Geometry: final body of the model. Coordinates: model frame, mm. Coordinates: 2 decimals unless noted, no trailing zeros. Write each loop counter-clockwise with the first axis right and the second up, starting at its lowest first coordinate (ties: lowest second). Pieces come first, ordered by that corner, then holes.
from build123d import *

# Parameters (mm, degrees)
SKETCH1_W              = 263.525
SKETCH1_H              = 50.8
BOSS_EXTRUDE1_DEPTH    = 1.143
F_10_CLEARANCE_HOLE1_D = 5.1054


with BuildPart() as part:
    # Sketch1 → Boss-Extrude1 (new, symmetric)
    with BuildSketch(Plane.XY):
        Rectangle(SKETCH1_W, SKETCH1_H)
    extrude(amount=BOSS_EXTRUDE1_DEPTH, both=True)

    # #10 Clearance Hole1 (through all)
    with Locations(Plane.XY.offset(1.143)):
        with Locations((-119.0625, 12.7), (-119.0625, -12.7), (-12.7, 12.7), (-12.7, -12.7), (12.7, -12.7), (12.7, 12.7), (119.0625, 12.7), (119.0625, -12.7)):
            Hole(F_10_CLEARANCE_HOLE1_D / 2)


solid = part.part
Item 1: Section A-A, the plane y = -12.7. Output: boundary loops of the cut face in (x, z).
Derived:
outline: (-131.76, -1.14) - (-121.62, -1.14) - (-121.62, 1.14) - (-131.76, 1.14) - close; (-116.51, -1.14) - (-15.25, -1.14) - (-15.25, 1.14) - (-116.51, 1.14) - close; (-10.15, -1.14) - (10.15, -1.14) - (10.15, 1.14) - (-10.15, 1.14) - close; (15.25, -1.14) - (116.51, -1.14) - (116.51, 1.14) - (15.25, 1.14) - close; (121.62, -1.14) - (131.76, -1.14) - (131.76, 1.14) - (121.62, 1.14) - close
Item 2: Material intervals for probe 1 along Y at (x, z) = (12.7, -0.3); probe 2 along X at (y, z) = (-12, 0.55), sorted ascending.
Derived:
probe 1: y = -25.4 to -15.25, -10.15 to 10.15, 15.25 to 25.4
probe 2: x = -131.76 to -121.52, -116.61 to -15.15, -10.25 to 10.25, 15.15 to 116.61, 121.52 to 131.76
Item 3: Section B-B, the plane x = 12.7. Output: boundary loops of the cut face in (y, z).
Derived:
outline: (-25.4, -1.14) - (-15.25, -1.14) - (-15.25, 1.14) - (-25.4, 1.14) - close; (-10.15, -1.14) - (10.15, -1.14) - (10.15, 1.14) - (-10.15, 1.14) - close; (15.25, -1.14) - (25.4, -1.14) - (25.4, 1.14) - (15.25, 1.14) - close
Item 4: Pin query (flat end, axial travel): pin 1 (4.5 mm diameter, centred on x = -12.7, y = -12.7, fed in from +Z). Return the tip coordinate at first contact, or that it passes through.
Derived:
pin 1: passes through
Item 5: Pull-direction query (X, two-part tool) for faces 1 (the cylindrical face through (119.62, -15.19, -0.02)), 2 (the flat face through (-2, 0, 1.143)), 3 (the cylindrical face through (-118.509, -15.192, -0.016)); classes: released by +X, released by -X, zero draft, split by the parting line, or undercut.
Derived:
face 1: undercut
face 2: zero draft
face 3: undercut
